Could you check a few things on this model? Use its own coordinates, in mm. A direction names the side the tool comes from. Coordinates: 2 decimals unless noted, no trailing zeros. Loops run counter-clockwise (first coordinate to the right, second up) from the corner with the lowest first, then second, coordinate; pieces in that order, holes last. Notation, with made-up numbers: (3.5, 29) -> (26.5, 29) arc R24 ccw to (26.5, 47) -> close; hole circle Ø3 at (-27, 17.5). An arc over 180 degrees is marked (long way). One line per question, with ' | ' between items.
```python
from build123d import *

# Parameters (mm, degrees)
SKETCH1_R           = 63.5
SKETCH1_R_2         = 42.926
SKETCH1_R_3         = 37.846
BOSS_EXTRUDE1_DEPTH = 19.05
SKETCH2_R           = 3.175
CUT_EXTRUDE1_DEPTH  = 92.800885072
CIRPATTERN1_COUNT   = 8
BOSS_EXTRUDE2_START = -25.4
SKETCH1_3_R         = 42.926
SKETCH1_3_R_2       = 37.846
BOSS_EXTRUDE2_DEPTH = 25.4
CUT_EXTRUDE2_START  = -13.97
SKETCH3_R           = 41.275
SKETCH3_R_2         = 37.846
CUT_EXTRUDE2_DEPTH  = 13.97
SKETCH4_W           = 2.697449546
SKETCH4_H           = 2.30839954
CUT_EXTRUDE3_DEPTH  = 101.201309872
SKETCH5_W           = 2.30839954
SKETCH5_H           = 7.62
CUT_EXTRUDE4_DEPTH  = 2.54
CIRPATTERN2_COUNT   = 18


with BuildPart() as part:
    # Sketch1 → Boss-Extrude1 (new body)
    # profile 1 of 2: a face of its own
    with BuildSketch(Plane(origin=(0, 0, 0), x_dir=(1, 0, 0), z_dir=(0, 1, 0))):
        with Locations(Location((0, 0, 0), (0, 0, 90))):
            Circle(SKETCH1_R)
        Circle(SKETCH1_R_2, mode=Mode.SUBTRACT)
    # profile 2 of 2: a face of its own
    with BuildSketch(Plane(origin=(0, 0, 0), x_dir=(1, 0, 0), z_dir=(0, 1, 0))):
        Circle(SKETCH1_R_2)
        with Locations(Location((0, 0, 0), (0, 0, 90))):
            Circle(SKETCH1_R_3, mode=Mode.SUBTRACT)
    extrude(amount=BOSS_EXTRUDE1_DEPTH)

    # Sketch2 → Cut-Extrude1 (cut, through all)
    with BuildSketch(Plane(origin=(0, 19.05, 0), x_dir=(1, 0, 0), z_dir=(0, 1, 0))):
        with Locations(Location((0, 55.88, 0), (0, 0, 270))):
            Circle(SKETCH2_R)
    cut_extrude1 = extrude(amount=-CUT_EXTRUDE1_DEPTH, mode=Mode.SUBTRACT)

    # CirPattern1: Cut-Extrude1 ×8 about axis
    cirpattern1_axis = Axis((0, 0, 0), (0, 1, 0))
    for i in range(1, CIRPATTERN1_COUNT):
        add(cut_extrude1.rotate(cirpattern1_axis, i * 360 / CIRPATTERN1_COUNT), mode=Mode.SUBTRACT)

    # Sketch1_3 → Boss-Extrude2 (add)
    with BuildSketch(Plane(origin=(0, 0, 0), x_dir=(1, 0, 0), z_dir=(0, 1, 0)).offset(BOSS_EXTRUDE2_START)):
        with Locations(Location((0, 0, 0), (0, 0, 270))):
            Circle(SKETCH1_3_R)
        with Locations(Location((0, 0, 0), (0, 0, 90))):
            Circle(SKETCH1_3_R_2, mode=Mode.SUBTRACT)
    extrude(amount=BOSS_EXTRUDE2_DEPTH)

    # Sketch3 → Cut-Extrude2 (cut)
    with BuildSketch(Plane(origin=(0, 19.05, 0), x_dir=(1, 0, 0), z_dir=(0, 1, 0)).offset(CUT_EXTRUDE2_START)):
        with Locations(Location((0, 0, 0), (0, 0, 270))):
            Circle(SKETCH3_R)
        with Locations(Location((0, 0, 0), (0, 0, 90))):
            Circle(SKETCH3_R_2, mode=Mode.SUBTRACT)
    extrude(amount=CUT_EXTRUDE2_DEPTH, mode=Mode.SUBTRACT)

    # Sketch4 → Cut-Extrude3 (cut, through all)
    with BuildSketch(Plane.XZ.offset(25.4)):
        with Locations((-39.422702208, 0)):
            Rectangle(SKETCH4_W, SKETCH4_H)
    cut_extrude3 = extrude(amount=-CUT_EXTRUDE3_DEPTH, mode=Mode.SUBTRACT)

    # Sketch5 → Cut-Extrude4 (cut)
    with BuildSketch(Plane.ZY.offset(38.073977435)):
        with Locations((0, 1.27)):
            Rectangle(SKETCH5_W, SKETCH5_H)
    cut_extrude4 = extrude(amount=-CUT_EXTRUDE4_DEPTH, mode=Mode.SUBTRACT)

    # CirPattern2: Cut-Extrude3, Cut-Extrude4 ×18 about axis
    cirpattern2_axis = Axis((0, 0, 0), (0, 1, 0))
    add([cut_extrude3.rotate(cirpattern2_axis, i * 360 / CIRPATTERN2_COUNT) for i in range(1, CIRPATTERN2_COUNT)], mode=Mode.SUBTRACT)
    add([cut_extrude4.rotate(cirpattern2_axis, i * 360 / CIRPATTERN2_COUNT) for i in range(1, CIRPATTERN2_COUNT)], mode=Mode.SUBTRACT)


solid = part.part
```
Q1. Imagine slicing it at B-B on x = 15. Write out the boundary of the cut face in (y, z), plus the area to 3 significant figures.
Values follow:
outline: (-25.4, -40.22) -> (0, -40.22) -> (0, -61.7) -> (19.05, -61.7) -> (19.05, -38.45) -> (5.08, -38.45) -> (5.08, -34.75) -> (-25.4, -34.75) -> close; (-25.4, 34.75) -> (5.08, 34.75) -> (5.08, 38.45) -> (19.05, 38.45) -> (19.05, 61.7) -> (0, 61.7) -> (0, 40.22) -> (-25.4, 40.22) -> close | area: 1,200 mm2
Q2. Please list where these lines run through material, in increasing order: L1, parallel to X at y = 10.5, z = 42; L2, parallel to Y at x = 35, z = -45; L3, parallel to X at y = 8, z = -54.5. Write a range as [from, to].
Values follow:
L1: x = [-47.63, -41.49], [-37.54, 37.54], [41.49, 47.63] | L2: y = [0, 19.05] | L3: x = [-32.59, -2.86], [2.86, 32.59]
Q3. We'd pull the mould along Z, two halves only. Please class faces 3 (the face through (36.58, 9.66, -38.3)), 4 (the face through (-39, -10, -1.154)), 5 (the face through (41.44, 19.05, -0.89)): released by +Z, released by -Z, zero draft, split by the parting line, or undercut.
Values follow:
face 3: undercut | face 4: undercut | face 5: zero draft
Q4. For pin 1 (2.5 mm diameter, centred on y = -13, z = 0.5, fed in from +X); pin 2 (0.5 mm diameter, centred on x = -29, z = -24, fed in from +Y); pin 3 (1 mm diameter, centred on x = -44, y = 10, fed in from -Z), each with a flat end and sliding along its axis, tell me the tip position at first contact or that it passes through.
Values follow:
pin 1: stops at x = 42.93 | pin 2: stops at y = -2.54 | pin 3: stops at z = -46.26
Q5. For faces 1 (the face through (-33.4, 5.08, 18.2)), 2 (the face through (0.14, 9.66, -59.05)), which set-ups out of +Z, -Z, +X, -X, +Y, -Y let a thin tool reach every point of the face, with its end or its side?
Values follow:
face 1: +Y | face 2: +Y, -Y
Q6. Imagine slicing it at A-A on z = -10. Write out the boundary of the cut face in (x, y).
Values follow:
outline: (-62.71, 0) -> (-41.74, 0) -> (-41.74, -25.4) -> (-36.5, -25.4) -> (-36.5, 5.08) -> (-40.05, 5.08) -> (-40.05, 19.05) -> (-62.71, 19.05) -> close; (36.5, -25.4) -> (41.74, -25.4) -> (41.74, 0) -> (62.71, 0) -> (62.71, 19.05) -> (40.05, 19.05) -> (40.05, 5.08) -> (36.5, 5.08) -> close
Q7. Imagine slicing it at C-C on y = -7. Give the number of separate pieces and of enclosed holes in the cut face, plus the area to 3 significant figures.
Values follow:
separate pieces: 1 | enclosed holes: 19 | area: 1,180 mm2
Q8. Imagine slicing it at D-D on z = -55.88. Write out the boundary of the cut face in (x, y) (3 decimals), plus the area to 3 significant figures.
Values follow:
outline: (-30.161, 0) -> (-3.175, 0) -> (-3.175, 19.05) -> (-30.161, 19.05) -> close; (3.175, 0) -> (30.161, 0) -> (30.161, 19.05) -> (3.175, 19.05) -> close | area: 1,030 mm2
